Check sheet for the modelled part. Datum: model origin and axes. Units: mm. A direction names the side the tool comes from. Round coordinates to 2 decimals unless told otherwise and drop trailing zeros. Order: outer loops, then holes, each group sorted by start corner. A loop starts at its lowest first (then second) coordinate and runs counter-clockwise, first axis right, second up. Notation, with made-up numbers: (-3, 89.25) -> (8, 89.25) arc R37 ccw to (8, 127.25) -> close; hole circle Ø9 at (49.5, -0.5). An arc over 180 degrees is marked (long way). Answer in a Markdown table with one row per item. Add a question column.
1. Material ranges on L1, parallel to X at y = 29, z = 11.5; L2, parallel to Z at x = -14, y = -22; L3, parallel to X at y = -2, z = 71.5, recorded low to high. Write a range as from..to.
2. Access from +Z, -Z, +X, -X, +Y, -Y to the whole of each face (thin tool, end or side, straight path). Record for faces 4 (the flat face through (-70.694, 2, 31)), 5 (the cylindrical face through (-52.006, 0.717, 80.241)), 6 (the flat face through (46, 21, 96.979)), 7 (the flat face through (76, 0, 61.895)).
3. Sectioned sample at B-B, the plane z = 74.5. Record the boundary of the cut face in (x, y).
4. Draft check along Y on faces 1 (the flat face through (-1, 3, 63.5)), 2 (the cylindrical face through (69.25, -41.88, 32.19)), 3 (the cylindrical face through (65.88, 0.7, 77.9)). Enter one of: +Y half, -Y half, draft (parallel to the pull), parting line (faces both ways), or undercut.
5. Sectioned sample at A-A, the plane y = 0. Record the boundary of the cut face in (x, z).
6. Depth check by flat-ended pin: P1, Ø4, axis at x = 51, y = -31.5, coming from the -Z side; P2, Ø10, axis at x = 37, y = 21.5, coming from the +Z side; P3, Ø6, axis at x = -8, z = 80, coming from the -Y side; P4, Ø4, axis at y = 24.5, z = 21.5, coming from the +X side. Enter the tip coordinate at first touch or a pass-through.
7. Sectioned sample at C-C, the plane z = 53. Record the boundary of the cut face in (x, y), then the cut area to 3 significant figures.
```python
from build123d import *

# Parameters (mm, degrees)
F0_W     = 141.3882523775
F0_H     = 86.8192017078
F1_DEPTH = 63.5
F2_R     = 28.5124697473
F3_DEPTH = 38.1
F4_R     = 16.3077330844
F5_DEPTH = 38.1
F6_W     = 16.9572941959
F6_H     = 35.0840575993
F8_R     = 5.08


with BuildPart() as f1:
    # F0 (on Top) → F1 (new body)
    with BuildSketch(Plane.XY):
        Rectangle(F0_W, F0_H)
    extrude(amount=F1_DEPTH)

    # F2 (on face) → F3 (join)
    with BuildSketch(Plane.XY.offset(63.5)):
        with Locations((-35.713609308, 0)):
            Circle(F2_R)
    extrude(amount=F3_DEPTH)

    # F4 (on face) → F5 (cut, through all)
    with BuildSketch(Plane.XY.offset(101.6)):
        with Locations((-35.713609308, 0)):
            Circle(F4_R)
    extrude(amount=-F5_DEPTH, mode=Mode.SUBTRACT)

    # F6 (on Front) → F7 (revolve)
    with BuildSketch(Plane.XZ):
        with Locations((25.4693310708, 79.4370155782)):
            Rectangle(F6_W, F6_H)
    revolve(axis=Axis((49.9209612608, 0, 63.9768075198), (0, 0, -1)))

    # F8
    f8_edges = [f1.edges().sort_by_distance(p)[0] for p in [
        (82.851239, 0, 96.979044),
        (-64.226079, 0, 101.6),
        (65.893944, 0, 96.979044),
        (0, -43.409601, 63.5),
        (70.694126, -43.409601, 31.75),
        (-70.694126, -43.409601, 31.75),
        (0, -43.409601, 0),
        (-52.021342, 0, 101.6),
    ]]
    fillet(f8_edges, radius=F8_R)


solid = f1.part
```
Answer key:
| question | item | result |
|---|---|---|
| 1 | L1 | x = -70.69..70.69 |
| 1 | L2 | z = 0..63.5 |
| 1 | L3 | x = -64.16..-51.9, -19.53..-7.27, 17.05..34.07, 65.77..82.79 |
| 2 | face 4 | +Z, -Z, -X, +Y, -Y |
| 2 | face 5 | +Z |
| 2 | face 6 | +Z, +X, +Y, -Y |
| 2 | face 7 | -Z, +X, +Y, -Y |
| 3 | outline | circle Ø57.02 at (-35.71, 0); circle Ø65.86 at (49.92, 0); hole circle Ø32.62 at (-35.71, 0); hole circle Ø31.95 at (49.92, 0) |
| 4 | face 1 | draft |
| 4 | face 2 | -Y half |
| 4 | face 3 | undercut |
| 5 | outline | (-70.69, 0) -> (70.69, 0) -> (70.69, 61.89) -> (82.85, 61.89) -> (82.85, 91.9) arc R5.08 ccw to (77.77, 96.98) -> (70.97, 96.98) arc R5.08 ccw to (65.89, 91.9) -> (65.89, 63.5) -> (33.95, 63.5) -> (33.95, 91.9) arc R5.08 ccw to (28.87, 96.98) -> (22.07, 96.98) arc R5.08 ccw to (16.99, 91.9) -> (16.99, 63.5) -> (-7.2, 63.5) -> (-7.2, 96.52) arc R5.08 ccw to (-12.28, 101.6) -> (-14.33, 101.6) arc R5.08 ccw to (-19.41, 96.52) -> (-19.41, 63.5) -> (-52.02, 63.5) -> (-52.02, 96.52) arc R5.08 ccw to (-57.1, 101.6) -> (-59.15, 101.6) arc R5.08 ccw to (-64.23, 96.52) -> (-64.23, 63.5) -> (-70.69, 63.5) -> close |
| 6 | P1 | stops at z = 0 |
| 6 | P2 | stops at z = 96.98 |
| 6 | P3 | stops at y = -14.22 |
| 6 | P4 | stops at x = 70.69 |
| 7 | outline | (-70.69, -38.33) arc R5.08 ccw to (-65.61, -43.41) -> (65.61, -43.41) arc R5.08 ccw to (70.69, -38.33) -> (70.69, 43.41) -> (-70.69, 43.41) -> close |
| 7 | area | 12,300 mm² |
